Input: part model. Units: mm. Frame: model coordinates. Give positions to 0.01 mm unless a question says otherwise; leave off trailing zeros. Loops run counter-clockwise (first coordinate to the right, second up) from the corner with the lowest first, then second, coordinate; pieces in that order, holes last. Notation, with made-up numbers: (54, 14) - (94, 14) arc R21 ccw to (94, 19) - close; hole circle Ø2 at (-29.75, 21.25). An arc over 180 degrees is marked (long way). Answer as a JSON object with one key per item and string values. Group by question number.
(1) Material intervals for L1, parallel to Y at x = -19, z = 10; L2, parallel to X at y = 4.25, z = 3.25; L3, parallel to Z at x = 9.5, y = 0.75, sorted ascending.
(2) Section query C-C (z = 12.75). Return loops of the section in (x, y), plus the area to 3 significant figures.
(3) Pin query (flat end, axial travel): P1, Ø8, axis at x = -25, z = 10.5, coming from the +Y side; P2, Ø0.8, axis at y = 5, z = 5.5, coming from the +X side. Return the tip coordinate at first contact, or that it passes through.
(4) Section query B-B (y = 3). Return loops of the section in (x, z), plus the area to 3 significant figures.
```python
from build123d import *

# Parameters (mm, degrees)
SKETCH2_W           = 100
SKETCH2_H           = 15
BOSS_EXTRUDE1_DEPTH = 4
FILLET4_R           = 2
BOSS_EXTRUDE4_DEPTH = 1.5


with BuildPart() as part:
    # Sketch2 → Boss-Extrude1 (new body)
    with BuildSketch(Plane(origin=(0, 0, 0), x_dir=(1, 0, 0), z_dir=(0, 1, 0))):
        with Locations((7.846153846, -6.346153846)):
            Rectangle(SKETCH2_W, SKETCH2_H)
    extrude(amount=BOSS_EXTRUDE1_DEPTH)

    # Fillet4
    fillet4_edges = [part.edges().sort_by_distance(p)[0] for p in [
        (7.846153846, 4, -1.153846154),
        (7.846153846, 0, -1.153846154),
        (7.846153846, 4, 13.846153846),
        (7.846153846, 0, 13.846153846),
    ]]
    fillet(fillet4_edges, radius=FILLET4_R - 0.0001)  # a hair under: the kernel refuses the full size

    # Sketch10 → Boss-Extrude4 (add)
    with BuildSketch(Plane(origin=(0, 4, 0), x_dir=(1, 0, 0), z_dir=(0, 1, 0))):
        with BuildLine():
            Line((53.846153846, -9.846153846), (53.846153846, -2.846153846))
            ThreePointArc((53.846153846, -2.846153846), (54.846153846, -1.846153846), (55.846153846, -2.846153846))
            Line((55.846153846, -2.846153846), (55.846153846, -9.846153846))
            ThreePointArc((55.846153846, -9.846153846), (54.846153846, -10.846153846), (53.846153846, -9.846153846))
        make_face()
    extrude(amount=BOSS_EXTRUDE4_DEPTH)

    # Loft6: read off the stored shape, not the designer's step
    # Loft6: loft between two sections, ruled curve by curve
    loft6_from = [
        Edge.make_bspline([(52.846153846, 5.5, 6.346153846), (52.846153846, 5.5, 6.893229755), (52.846153846, 5.5, 7.987381572), (52.846153846, 5.5, 9.172470024), (52.846153846, 5.5, 10.062777988), (52.916794739, 5.5, 10.520533365), (53.297264612, 5.5, 11.19493708), (53.970100399, 5.5, 11.713677023), (54.846153846, 5.5, 11.912823977), (55.722207294, 5.5, 11.713677023), (56.395043081, 5.5, 11.19493708), (56.775512954, 5.5, 10.520533365), (56.846153846, 5.5, 10.062777988), (56.846153846, 5.5, 9.172470024), (56.846153846, 5.5, 7.987381572), (56.846153846, 5.5, 6.346153846), (56.846153846, 5.5, 4.70492612), (56.846153846, 5.5, 3.519837669), (56.846153846, 5.5, 2.629529705), (56.775512954, 5.5, 2.171774328), (56.395043081, 5.5, 1.497370612), (55.722207294, 5.5, 0.97863067), (54.846153846, 5.5, 0.779483716), (53.970100399, 5.5, 0.97863067), (53.297264612, 5.5, 1.497370612), (52.916794739, 5.5, 2.171774328), (52.846153846, 5.5, 2.629529705), (52.846153846, 5.5, 3.519837669), (52.846153846, 5.5, 4.70492612), (52.846153846, 5.5, 5.799077937), (52.846153846, 5.5, 6.346153846)], [0.347848884, 0.347848884, 0.347848884, 0.347848884, 0.423924442, 0.5, 0.5, 0.524462221, 0.548924442, 0.573386663, 0.597848884, 0.622311105, 0.646773326, 0.671235547, 0.695697768, 0.695697768, 0.771773326, 0.847848884, 0.923924442, 1, 1, 1.024462221, 1.048924442, 1.073386663, 1.097848884, 1.122311105, 1.146773326, 1.171235547, 1.195697768, 1.195697768, 1.271773326, 1.347848884, 1.347848884, 1.347848884, 1.347848884], 3),
    ]
    loft6_to = [
        Edge.make_bspline([(53.846153846, 6.5, 6.346153846), (53.846153846, 6.5, 6.970863619), (53.846153846, 6.5, 8.220283163), (53.846153846, 6.5, 9.3318023), (53.846153846, 6.5, 10.011544432), (53.92463889, 6.5, 10.301418233), (54.169662015, 6.5, 10.614768288), (54.490600847, 6.5, 10.803946654), (54.846153846, 6.5, 10.867265337), (55.201706845, 6.5, 10.803946654), (55.522645677, 6.5, 10.614768288), (55.767668802, 6.5, 10.301418233), (55.846153846, 6.5, 10.011544432), (55.846153846, 6.5, 9.3318023), (55.846153846, 6.5, 8.220283163), (55.846153846, 6.5, 6.346153846), (55.846153846, 6.5, 4.472024529), (55.846153846, 6.5, 3.360505393), (55.846153846, 6.5, 2.68076326), (55.767668802, 6.5, 2.390889459), (55.522645677, 6.5, 2.077539404), (55.201706845, 6.5, 1.888361038), (54.846153846, 6.5, 1.825042355), (54.490600847, 6.5, 1.888361038), (54.169662015, 6.5, 2.077539404), (53.92463889, 6.5, 2.390889459), (53.846153846, 6.5, 2.68076326), (53.846153846, 6.5, 3.360505393), (53.846153846, 6.5, 4.472024529), (53.846153846, 6.5, 5.721444074), (53.846153846, 6.5, 6.346153846)], [0.347848884, 0.347848884, 0.347848884, 0.347848884, 0.423924442, 0.5, 0.5, 0.524462221, 0.548924442, 0.573386663, 0.597848884, 0.622311105, 0.646773326, 0.671235547, 0.695697768, 0.695697768, 0.771773326, 0.847848884, 0.923924442, 1, 1, 1.024462221, 1.048924442, 1.073386663, 1.097848884, 1.122311105, 1.146773326, 1.171235547, 1.195697768, 1.195697768, 1.271773326, 1.347848884, 1.347848884, 1.347848884, 1.347848884], 3),
    ]
    loft6 = Solid(Shell([*[Face.make_surface_from_curves(loft6_from[k], loft6_to[k]) for k in range(1)], Face(Wire(loft6_from)), Face(Wire(loft6_to))]))
    add(loft6)


solid = part.part
```
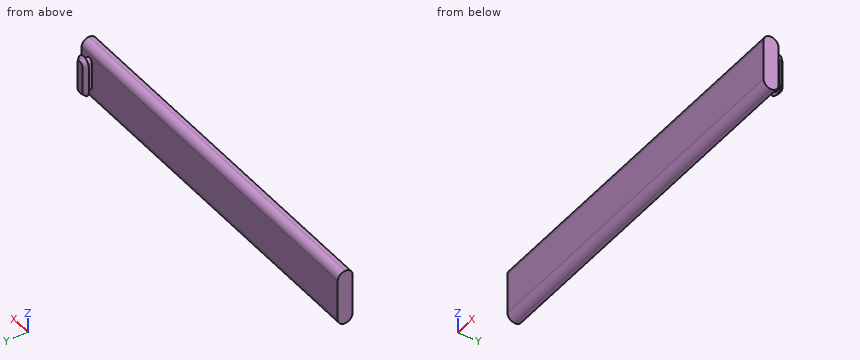
Recorded:
{
 "1": {"L1": "y = 0 to 4", "L2": "x = 53.85 to 55.85", "L3": "z = -0.72 to 13.41"},
 "2": {"outline": "(-42.15, 0.22) - (57.85, 0.22) - (57.85, 3.78) - (-42.15, 3.78) - close", "area": "357 mm^2"},
 "3": {"P1": "stops at y = 4", "P2": "stops at x = 55.85"},
 "4": {"outline": "(-42.15, -0.89) - (57.85, -0.89) - (57.85, 13.58) - (-42.15, 13.58) - close", "area": "1,450 mm^2"}
}
